```python
from build123d import *

# Parameters (mm, degrees)
PAH1_SIZE = 0.5


with BuildPart() as part:
    # Çizim1 → Döndür1 (revolve)
    with BuildSketch(Plane.XY, mode=Mode.PRIVATE) as d_nd_r1_sk:
        Polygon((0, 0), (0, 4), (35, 4), (50.491933385, 8), (129.303061543, 8), (144, 5), (154.5, 5), (154.5, 3.5), (198.5, 3.5), (198.5, 0), align=None)
    revolve(d_nd_r1_sk.sketch.rotate(Axis((0, 0, 0), (1, 0, 0)), 90), axis=Axis((0, 0, 0), (1, 0, 0)))

    # Pah1
    pah1_edges = [part.edges().sort_by_distance(p)[0] for p in [
        (0, 0, -4),
    ]]
    chamfer(pah1_edges, length=PAH1_SIZE)


solid = part.part
```
CAD build for the part. Positions are in the model's coordinates, mm. A direction names the side the tool comes from. Coordinates: 2 decimals unless noted, no trailing zeros. Order: outer loops, then holes, each group sorted by start corner. A loop starts at its lowest first (then second) coordinate and runs counter-clockwise, first axis right, second up.
(1) Saw through at D-D, the plane x = 84.5. Write the cut outline in (y, z), and give its area (3 significant figures).
Solution:
outline: circle Ø16 at (0, 0)
area: 201 mm2
(2) Saw through at A-A, the plane y = 0. Write the cut outline in (x, z), and give its area (3 significant figures).
Solution:
outline: (0, -3.5) - (0.5, -4) - (35, -4) - (50.49, -8) - (129.3, -8) - (144, -5) - (154.5, -5) - (154.5, -3.5) - (198.5, -3.5) - (198.5, 3.5) - (154.5, 3.5) - (154.5, 5) - (144, 5) - (129.3, 8) - (50.49, 8) - (35, 4) - (0.5, 4) - (0, 3.5) - close
area: 2,330 mm2
(3) Which spindle directions (+Z, -Z, +X, -X, +Y, -Y) get a long thin tool onto all of the face, cutting with end or side? Do faces 1 (the face through (90.45, 7.81, -1.73)), 2 (the face through (149, 0, -5)), 3 (the face through (17.992, 3.905, -0.867)). Say none if no direction does.
Solution:
face 1: +X, -X
face 2: +X
face 3: -X
(4) Saw through at C-C, the plane x = 164. Write the cut outline in (y, z), and give its area (3 significant figures).
Solution:
outline: circle Ø7 at (0, 0)
area: 38.5 mm2
(5) Pin check, flat tips, straight feed: pin 1 Ø6 at (x, y) = (170.5, -5) entering from +Z; pin 2 Ø8 at (x, z) = (153.5, 1.5) entering from -Y. Stop position of each tip, or through.
Solution:
pin 1: stops at z = 2.87
pin 2: stops at y = -5
(6) Drill centre lines: L1, parallel to Z at x = 71.5, y = -0.5; L2, parallel to Y at x = 185.5, z = -0.5; L3, parallel to Z at x = 172.5, y = -0.25. Where is each one in solid material? Low to high.
Solution:
L1: z = -7.98 to 7.98
L2: y = -3.46 to 3.46
L3: z = -3.49 to 3.49
